CAD build for the part. Positions are in the model's coordinates, mm. A direction names the side the tool comes from. Give positions to 0.01 mm unless a question says otherwise; leave off trailing zeros. Loops run counter-clockwise (first coordinate to the right, second up) from the corner with the lowest first, then second, coordinate; pieces in that order, holes last. Notation, with made-up numbers: (-24, 59.5) -> (14, 59.5) arc R30 ccw to (14, 96.5) -> close; hole circle Ø1 at (78.5, 25). An arc over 180 degrees is marked (long way). Use one line per item in the form item = value.
```python
from build123d import *

# Parameters (mm, degrees)
MODEL_W         = 13.9993
MODEL_H         = 13.9993
EXTRUDE_1_DEPTH = 1.5
EXTRUDE_START   = 3.5
EXTRUDE_2_DEPTH = 3.5
CHAMFER_1_SIZE  = 2
EXTRUDE_START_2 = 1
EXTRUDE_3_DEPTH = 1


with BuildPart() as part:
    # Model → 凸台-拉伸1 (new body)
    with BuildSketch(Plane.XY):
        with BuildLine():
            Line((45.999313773, 49.434568323), (-44.302972349, 49.434568323))
            ThreePointArc((-44.302972349, 49.434568323), (-49.252719817, 47.384315792), (-51.302972349, 42.434568323))
            Line((-51.302972349, 42.434568323), (-51.302972349, -29.48760905))
            ThreePointArc((-51.302972349, -29.48760905), (-44.859321535, -45.043958236), (-29.302972349, -51.48760905))
            Line((-29.302972349, -51.48760905), (48.628680412, -51.48760905))
            Line((48.628680412, -51.48760905), (48.628680412, 9.328079248))
            Line((48.628680412, 9.328079248), (52.178865693, 12.878264529))
            Line((52.178865693, 12.878264529), (52.178865693, 43.255016404))
            Line((52.178865693, 43.255016404), (45.999313773, 49.434568323))
        make_face()
        Polygon((37.658208977, 36.530428762), (26.934123004, 27.531852177), (35.932699588, 16.807766205), (46.656785561, 25.806342789), align=None, mode=Mode.SUBTRACT)
        Polygon((13.937335593, 43.369798663), (4.938759009, 32.64571269), (15.662844981, 23.647136106), (24.661421566, 34.371222079), align=None, mode=Mode.SUBTRACT)
        Polygon((-11.724299854, 43.912488191), (-20.722876438, 33.188402219), (-9.998790465, 24.189825635), (-1.000213881, 34.913911607), align=None, mode=Mode.SUBTRACT)
        Polygon((-36.782315633, 39.237800689), (-45.780892217, 28.513714717), (-35.056806244, 19.515138133), (-26.05822966, 30.239224105), align=None, mode=Mode.SUBTRACT)
        Polygon((34.81841009, 8.16776686), (22.000122493, 13.79554649), (16.372342863, 0.977258893), (29.19063046, -4.650520737), align=None, mode=Mode.SUBTRACT)
        Polygon((3.45628169, 26.205455431), (-5.542294894, 15.481369459), (5.181791078, 6.482792875), (14.180367663, 17.206878847), align=None, mode=Mode.SUBTRACT)
        with Locations((17.862828836, -39.410351083)):
            Rectangle(MODEL_W, MODEL_H, mode=Mode.SUBTRACT)
        with Locations((36.913128836, -39.410351083)):
            Rectangle(MODEL_W, MODEL_H, mode=Mode.SUBTRACT)
        Polygon((20.363631661, -17.43145013), (18.837631661, -17.43145013), (18.837631661, -14.20145013), (17.112631661, -14.20145013), (17.112631661, -13.28205013), (13.813631661, -13.28205013), (13.813631661, -14.20145013), (12.086831661, -14.20145013), (12.086831661, -17.43145013), (11.262731661, -17.43145013), (11.262731661, -20.23165013), (12.086831661, -20.23165013), (12.086831661, -26.50175013), (13.813631661, -26.50175013), (13.813631661, -27.48155013), (17.112631661, -27.48155013), (17.112631661, -26.50175013), (18.837631661, -26.50175013), (18.837631661, -22.03145013), (20.363631661, -22.03145013), (20.363631661, -26.73185013), (34.362631661, -26.73185013), (34.362631661, -22.03145013), (35.888631661, -22.03145013), (35.888631661, -26.50175013), (37.613631661, -26.50175013), (37.613631661, -27.48155013), (40.912631661, -27.48155013), (40.912631661, -26.50175013), (42.637631661, -26.50175013), (42.637631661, -20.23165013), (43.463631661, -20.23165013), (43.463631661, -17.43145013), (42.637631661, -17.43145013), (42.637631661, -14.20145013), (40.912631661, -14.20145013), (40.912631661, -13.28205013), (37.613631661, -13.28205013), (37.613631661, -14.20145013), (35.888631661, -14.20145013), (35.888631661, -17.43145013), (34.362631661, -17.43145013), (34.362631661, -12.73245013), (20.363631661, -12.73245013), align=None, mode=Mode.SUBTRACT)
        with Locations((-38.908302282, 3.381462696)):
            Rectangle(MODEL_W, MODEL_H, mode=Mode.SUBTRACT)
        with Locations((-19.758451091, 3.325597175)):
            Rectangle(MODEL_W, MODEL_H, mode=Mode.SUBTRACT)
        with Locations((-10.932627063, -26.471328106)):
            Rectangle(MODEL_W, MODEL_H, mode=Mode.SUBTRACT)
    extrude(amount=EXTRUDE_1_DEPTH)

    # 草图1 → 凸台-拉伸2 (add)
    with BuildSketch(Plane(origin=(0, 0, 0), x_dir=(-1, 0, 0), z_dir=(0, 0, -1)).offset(EXTRUDE_START)):
        with BuildLine():
            Line((51.302972349, -29.48760905), (51.302972349, 42.434568323))
            ThreePointArc((51.302972349, 42.434568323), (49.252719817, 47.384315792), (44.302972349, 49.434568323))
            Line((44.302972349, 49.434568323), (-45.999313773, 49.434568323))
            Line((-45.999313773, 49.434568323), (-52.178865693, 43.255016404))
            Line((-52.178865693, 43.255016404), (-52.178865693, 12.878264529))
            Line((-52.178865693, 12.878264529), (-48.628680412, 9.328079248))
            Line((-48.628680412, 9.328079248), (-48.628680412, -51.48760905))
            Line((-48.628680412, -51.48760905), (29.302972349, -51.48760905))
            ThreePointArc((29.302972349, -51.48760905), (44.859321535, -45.043958236), (51.302972349, -29.48760905))
        make_face()
        with BuildLine():
            Line((44.302972349, 46.434568323), (-44.756673086, 46.434568323))
            Line((-44.756673086, 46.434568323), (-49.178865693, 42.012375717))
            Line((-49.178865693, 42.012375717), (-49.178865693, 14.120905216))
            Line((-49.178865693, 14.120905216), (-45.628680412, 10.570719935))
            Line((-45.628680412, 10.570719935), (-45.628680412, -48.48760905))
            Line((-45.628680412, -48.48760905), (29.302972349, -48.48760905))
            ThreePointArc((29.302972349, -48.48760905), (42.738001191, -42.922637892), (48.302972349, -29.48760905))
            Line((48.302972349, -29.48760905), (48.302972349, 42.434568323))
            ThreePointArc((48.302972349, 42.434568323), (47.131399474, 45.262995448), (44.302972349, 46.434568323))
        make_face(mode=Mode.SUBTRACT)
    extrude(amount=-EXTRUDE_2_DEPTH)

    # 倒角1
    chamfer_1_edges = [part.edges().sort_by_distance(p)[0] for p in [
        (48.628680412, -51.48760905, -1),
    ]]
    chamfer(chamfer_1_edges, length=CHAMFER_1_SIZE)

    # 草图2 → 凸台-拉伸3 (add)
    with BuildSketch(Plane(origin=(0, 0, -3.5), x_dir=(-1, 0, 0), z_dir=(0, 0, -1)).offset(EXTRUDE_START_2)):
        with BuildLine():
            Line((-52.178865693, 43.255016404), (-50.278865693, 42.468010635))
            Line((-50.278865693, 42.468010635), (-50.278865693, 13.665270298))
            Line((-50.278865693, 13.665270298), (-46.728680412, 10.115085017))
            Line((-46.728680412, 10.115085017), (-46.728680412, -48.700603281))
            Line((-46.728680412, -48.700603281), (-45.841674643, -49.58760905))
            Line((-45.841674643, -49.58760905), (29.302972349, -49.58760905))
            ThreePointArc((29.302972349, -49.58760905), (43.515818651, -43.700455352), (49.402972349, -29.48760905))
            Line((49.402972349, -29.48760905), (49.402972349, 42.434568323))
            ThreePointArc((49.402972349, 42.434568323), (47.909216933, 46.040812908), (44.302972349, 47.534568323))
            Line((44.302972349, 47.534568323), (-45.212308005, 47.534568323))
            Line((-45.212308005, 47.534568323), (-45.999313773, 49.434568323))
            Line((-45.999313773, 49.434568323), (44.302972349, 49.434568323))
            ThreePointArc((44.302972349, 49.434568323), (49.252719817, 47.384315792), (51.302972349, 42.434568323))
            Line((51.302972349, 42.434568323), (51.302972349, -29.48760905))
            ThreePointArc((51.302972349, -29.48760905), (44.859321535, -45.043958236), (29.302972349, -51.48760905))
            Line((29.302972349, -51.48760905), (-46.628680412, -51.48760905))
            Line((-46.628680412, -51.48760905), (-48.628680412, -49.48760905))
            Line((-48.628680412, -49.48760905), (-48.628680412, 9.328079248))
            Line((-48.628680412, 9.328079248), (-52.178865693, 12.878264529))
            Line((-52.178865693, 12.878264529), (-52.178865693, 43.255016404))
        make_face()
    extrude(amount=-EXTRUDE_3_DEPTH)


solid = part.part
```
1. Mould opens along X. For faces 5 (the cylindrical face through (-42.59, -43.07, -1.77)), 6 (the cylindrical face through (-45, -44.9, -1.5)), 7 (the flat face through (0, 0, 1.5)), 8 (the flat face through (52.179, 28, -2)) say: pulls with the +X half, pulls with the -X half, needs draft (parallel to the pull), parting line crosses it, or undercut.
Result sheet:
face_5 = undercut
face_6 = pulls with the -X half
face_7 = needs draft
face_8 = pulls with the +X half
2. Cut at B-B, the plane z = -2.5. Write the cut outline in (x, y), then the cut area to 3 significant figures.
Result sheet:
outline = (-51.3, -29.49) arc R22 ccw to (-29.3, -51.49) -> (46.63, -51.49) -> (48.63, -49.49) -> (48.63, 9.33) -> (52.18, 12.88) -> (52.18, 43.26) -> (46, 49.43) -> (-44.3, 49.43) arc R7 ccw to (-51.3, 42.43) -> close; hole (-48.3, -29.49) arc R19 ccw to (-29.3, -48.49) -> (45.63, -48.49) -> (45.63, 10.57) -> (49.18, 14.12) -> (49.18, 42.01) -> (44.76, 46.43) -> (-44.3, 46.43) arc R4 ccw to (-48.3, 42.43) -> close
area = 1,140 mm^2
3. Drop a flat-ended pin along its axis: P1, Ø0.8, axis at y = -23.5, z = 0.5, coming from the +X side. Give the stop position or say it passes through.
Result sheet:
P1 = 48.63
4. Cut at C-C, the plane x = 9. Write the cut outline in (y, z), then the cut area to 3 significant figures.
Result sheet:
outline = (-51.49, -4.5) -> (-49.59, -4.5) -> (-49.59, -3.5) -> (-48.49, -3.5) -> (-48.49, 0) -> (11.03, 0) -> (11.03, 1.5) -> (-51.49, 1.5) -> close; (21.55, 0) -> (29.24, 0) -> (29.24, 1.5) -> (21.55, 1.5) -> close; (37.49, 0) -> (46.43, 0) -> (46.43, -3.5) -> (47.53, -3.5) -> (47.53, -4.5) -> (49.43, -4.5) -> (49.43, 1.5) -> (37.49, 1.5) -> close
area = 148 mm^2
5. Cut at D-D, the plane x = -42.5. Write the cut outline in (y, z).
Result sheet:
outline = (-47.09, -4.5) -> (-44.65, -4.5) -> (-44.65, -3.5) -> (-43.16, -3.5) -> (-43.16, 0) -> (-3.62, 0) -> (-3.62, 1.5) -> (-47.09, 1.5) -> close; (10.38, 0) -> (25.76, 0) -> (25.76, 1.5) -> (10.38, 1.5) -> close; (32.42, 0) -> (46.43, 0) -> (46.43, -3.5) -> (47.53, -3.5) -> (47.53, -4.5) -> (49.43, -4.5) -> (49.43, 1.5) -> (32.42, 1.5) -> close
6. Cut at A-A, the plane x = -16. Write the cut outline in (y, z).
Result sheet:
outline = (-51.49, -4.5) -> (-49.59, -4.5) -> (-49.59, -3.5) -> (-48.49, -3.5) -> (-48.49, 0) -> (-33.47, 0) -> (-33.47, 1.5) -> (-51.49, 1.5) -> close; (-19.47, 0) -> (-3.67, 0) -> (-3.67, 1.5) -> (-19.47, 1.5) -> close; (10.33, 0) -> (29.23, 0) -> (29.23, 1.5) -> (10.33, 1.5) -> close; (38.82, 0) -> (46.43, 0) -> (46.43, -3.5) -> (47.53, -3.5) -> (47.53, -4.5) -> (49.43, -4.5) -> (49.43, 1.5) -> (38.82, 1.5) -> close
7. Tool access for faces 1 (the flat face through (49.046, 46.388, -1.035)), 2 (the flat face through (48.529, 11.915, -4.007)), 3 (the flat face through (0, 0, 0)), 4 (the flat face through (22.7, -1.8, 0.7)): list every direction of +Z, -Z, +X, -X, +Y, -Y with a clear straight run to the whole face (end or side of a thin tool).
Result sheet:
face_1 = +Z, -Z, +X, +Y
face_2 = -Z, +Y
face_3 = -Z
face_4 = +Z, -Z
8. Drill centre lines: line 1 (X direction, y = -21, z = 0.4); line 2 (Y direction, x = 43.5, z = -1.55); line 3 (X direction, y = -23.5, z = 0.7). Where is each one in solid material? Low to high.
Result sheet:
line_1 = -51.3 to -17.93, -3.93 to 12.09, 42.64 to 48.63
line_2 = -51.49 to -48.49, 46.43 to 49.43
line_3 = -51.3 to -17.93, -3.93 to 12.09, 18.84 to 20.36, 34.36 to 35.89, 42.64 to 48.63
